Autodesk Inventor part; units mm, degrees
ref_plane "YZ Plane" through (0, 0, 0) normal (1, 0, 0) x (0, 1, 0)
ref_plane "XZ Plane" through (0, 0, 0) normal (0, 1, 0) x (-1, 0, 0)
ref_plane "XY Plane" through (0, 0, 0) normal (0, 0, 1) x (1, 0, 0)
sketch "Sketch1" plane through (0, 0, 0) normal (1, 0, 0) x (0, 1, 0)
  line L0 (13.7592, -3.5232) -> (-6.0382, 7.9068) construction
  line L1 (-6.0382, 7.9068) -> (13.7592, 19.3368) construction
  line L2 (13.7592, 19.3368) -> (13.7592, -3.5232) construction
  circle A0 centre (13.7592, 19.3368) radius 3.175
  circle A1 centre (13.7592, -3.5232) radius 3.175
  circle A2 centre (-6.0382, 7.9068) radius 3.175
  line L3 (-6.0382, 7.9068) -> (-15.5632, 7.9068) construction
  line L4 (-10.8007, 10.6565) -> (13.7592, 24.8361)
  line L5 (18.5217, 22.0865) -> (18.5217, -6.2728)
  line L6 (13.7592, -9.0224) -> (-10.8007, 5.1572)
  arc A3 (18.5217, 22.0865) -> (13.7592, 24.8361) centre (15.3467, 22.0865) ccw
  arc A4 (-10.8007, 10.6565) -> (-10.8007, 5.1572) centre (-9.2132, 7.9068) ccw
  arc A5 (13.7592, -9.0224) -> (18.5217, -6.2728) centre (15.3467, -6.2728) ccw
  point P0 (7.1601, 7.9068)
  point P1 (7.1601, 7.9068)
  point P2 (18.5217, 27.5857)
  point P3 (18.5217, -11.7721)
  dimension "d7" = 22.86
  dimension "d8" = 6.35
  dimension "d9" = 6.35
  dimension "d10" = 6.35
  dimension "d11" = 9.525
  dimension "d12" = 3.175
extrude "Extrusion1" add sketch "Sketch1" along normal blind 3.175
properties part number "arm4_3"
Work out the finished part from the listing and answer in its coordinate system (mm). Round coordinates to 2 decimals unless told otherwise and drop trailing zeros. Write each loop counter-clockwise with the first axis right and the second up, starting at its lowest first coordinate (ties: lowest second). Pieces come first, ordered by that corner, then holes. Notation, with made-up numbers: (61.25, -6) -> (111.25, -6) arc R33 ccw to (111.25, 31) -> close; hole circle Ø4 at (79, 40). An arc over 180 degrees is marked (long way). Answer as CSV lines item,"result". Start each with the question number.
(1) The part is cut by section A-A, the plane z = -2.5. Give the vertices of the cut face in (x, y) (3 decimals), then the cut area to 3 significant figures.
(2) The mould has two halves that part along Z. Classify faces 1 (the flat face through (1.57, 1.65, -2.03)), 2 (the cylindrical face through (1.565, 16.692, -2.307)), 3 (the flat face through (3.175, 6, 8)): +Z half, -Z half, draft (parallel to the pull), parting line (faces both ways), or undercut.
(3) The part is cut by section B-B, the plane y = 12. Give the vertices of the cut face in (x, z) (3 decimals).
(4) The part is cut by section C-C, the plane x = 1. Give the number of separate pieces and of enclosed holes in the cut face, then the cut area to 3 significant figures.
(5) Find the intervals of material crossed by probe 1 along Z at (x, y) = (2.45, 11.5); probe 2 along Y at (x, z) = (0.6, 8); probe 3 along Z at (x, y) = (1.2, 12), in increasing order.
(6) The part is cut by section D-D, the plane y = -5. Give the vertices of the cut face in (x, z) (3 decimals).
Output values:
1,outline,"(0, 2.462) -> (3.175, 2.462) -> (3.175, 10.754) -> (0, 10.754) -> close; (0, 16.765) -> (3.175, 16.765) -> (3.175, 18.522) -> (0, 18.522) -> close"
1,area,"31.9 mm²"
2,face 1,"-Z half"
2,face 2,"undercut"
2,face 3,"draft"
3,outline,"(0, -8.007) -> (3.175, -8.007) -> (3.175, -6.166) -> (0, -6.166) -> close; (0, -0.88) -> (3.175, -0.88) -> (3.175, 16.694) -> (0, 16.694) -> close; (0, 21.98) -> (3.175, 21.98) -> (3.175, 23.82) -> (0, 23.82) -> close"
4,separate pieces,"1"
4,enclosed holes,"3"
4,area,"555 mm²"
5,probe 1,"z = -7.72 to -5.75, -1.29 to 17.11, 21.57 to 23.53"
5,probe 2,"y = -12.39 to -9.21, -2.86 to 18.52"
5,probe 3,"z = -8.01 to -6.17, -0.88 to 16.69, 21.98 to 23.82"
6,outline,"(0, 1.808) -> (3.175, 1.808) -> (3.175, 4.906) -> (0, 4.906) -> close; (0, 10.907) -> (3.175, 10.907) -> (3.175, 14.006) -> (0, 14.006) -> close"
